The listing builds one solid part. Answer for the finished solid, in the listing's coordinates (mm). A direction names the side the tool comes from. Round coordinates to 2 decimals unless told otherwise and drop trailing zeros. Write each loop counter-clockwise with the first axis right and the second up, starting at its lowest first coordinate (ties: lowest second). Pieces come first, ordered by that corner, then holes. Notation, with made-up numbers: (78, -24) - (118, -24) arc R20 cw to (118, -11) - close; hole circle Ø2 at (-29.5, 42.25). An arc over 180 degrees is marked (long way). Return JSON: item names as keys, results as strings. Group by question number.
(1) Determine the mould class of faces 6 (the cylindrical face through (-3.32, -5.98, -0.03)), 7 (the flat face through (0, -2, -2)), 8 (the cylindrical face through (1.805, -6.618, -0.028)) for opening direction X: +X half, -X half, draft (parallel to the pull), parting line (faces both ways), or undercut.
(2) Each of these flat-tipped pins is pushed along its axis until it touches: pin 1 (1 mm diameter, centred on y = 0.5, z = 0, fed in from +X); pin 2 (1 mm diameter, centred on x = -2.5, z = 1, fed in from -Y); pin 3 (1 mm diameter, centred on y = -2, z = 1, fed in from -X). Where does it stop, or does it pass through?
(3) Which of the six approach directions +Z, -Z, +X, -X, +Y, -Y give full straight-line access (tool end or side, diameter ignored) to faces 1 (the cylindrical face through (4.66, 5.015, -0.028)), 2 (the cylindrical face through (2.6, 6.85, 0.03)), 3 (the cylindrical face through (-5.534, -1.997, 0.028)), 4 (the cylindrical face through (2.822, 5.177, -0.028)), 5 (the cylindrical face through (-0.16, -6.84, -0.03))?
(4) Section A-A, the plane x = -2.75 is taken. Write down the section's boundary in (y, z), then the cut area to 3 significant figures.
(5) Find the intervals of material crossed by line 1 along X through (y, z) = (0, 0.3); line 2 along Y through (x, z) = (-6.5, -1.45); line 3 along X through (y, z) = (5.5, 0.35), in increasing order. Write a range as [from, to].
```python
from build123d import *

# Parameters (mm, degrees)
SKETCH1_R                = 7.326923077
BLANK_DISK_DEPTH         = 2
GEAR_TOOTH_CUT_DEPTH     = 12.107097013
GEAR_START               = -2.000000064
GEAR_TEETH_REVOLVE_DEPTH = 4.000000128
SKETCH4_R                = 0.75
HUB_EXTRUDE_DEPTH        = 0.635
HEX_BORE_CUT_DEPTH       = 12.099256278
HEX_BORE_CUT_DEPTH_BACK  = 12.099256278


# Read off the part's stored shape, not the designer's step: GEAR TEETH REVOLVE
with BuildPart() as part:
    # Sketch1 → BLANK DISK (new, symmetric)
    with BuildSketch(Plane.XY):
        Circle(SKETCH1_R)
    extrude(amount=BLANK_DISK_DEPTH, both=True)

    # Sketch2 → GEAR TOOTH CUT (cut, through all)
    with BuildSketch(Plane.XY.offset(2.000000064)):
        with BuildLine():
            ThreePointArc((-6.69170719, -2.984100644), (-7.114016008, -1.753447463), (-7.311993171, -0.467501495))
            ThreePointArc((-7.311993171, -0.467501495), (-6.820672406, -0.660972702), (-6.303462426, -0.767373077))
            ThreePointArc((-6.303462426, -0.767373077), (-5.834645763, -0.80350314), (-5.364440786, -0.802189535))
            ThreePointArc((-5.364440786, -0.802189535), (-5.140559328, -0.873425337), (-5.015496519, -1.072314102))
            ThreePointArc((-5.015496519, -1.072314102), (-4.979811206, -1.227413224), (-4.939330826, -1.381330469))
            ThreePointArc((-4.939330826, -1.381330469), (-4.957640225, -1.615557309), (-5.122772484, -1.782676381))
            ThreePointArc((-5.122772484, -1.782676381), (-5.539728776, -2.000028389), (-5.938054838, -2.249889939))
            ThreePointArc((-5.938054838, -2.249889939), (-6.346574811, -2.584462254), (-6.69170719, -2.984100644))
        make_face()
    extrude(amount=-GEAR_TOOTH_CUT_DEPTH, mode=Mode.SUBTRACT)

    # GEAR TEETH REVOLVE outline → GEAR TEETH REVOLVE (cut)
    with BuildSketch(Plane.XY.offset(GEAR_START)):
        with BuildLine():
            ThreePointArc((-6.257189634, -3.812004676), (-5.484280674, -4.858648706), (-4.538431736, -5.752081287))
            ThreePointArc((-4.538431736, -5.752081287), (-4.418553413, -5.237828053), (-4.212310448, -4.751730284))
            ThreePointArc((-4.212310448, -4.751730284), (-3.975726688, -4.345377518), (-3.707538741, -3.959152621))
            ThreePointArc((-3.707538741, -3.959152621), (-3.638985493, -3.734435245), (-3.731623965, -3.518528876))
            ThreePointArc((-3.731623965, -3.518528876), (-3.838996472, -3.401054095), (-3.942672404, -3.280304435))
            ThreePointArc((-3.942672404, -3.280304435), (-4.145838239, -3.162316765), (-4.377180353, -3.203283496))
            ThreePointArc((-4.377180353, -3.203283496), (-4.79291572, -3.422961784), (-5.224822737, -3.608840169))
            ThreePointArc((-5.224822737, -3.608840169), (-5.73223615, -3.754986778), (-6.257189634, -3.812004676))
        make_face()
        with BuildLine():
            ThreePointArc((-3.76893936, -6.283223524), (-2.59816273, -6.850792084), (-1.345456266, -7.202329428))
            ThreePointArc((-1.345456266, -7.202329428), (-1.478294676, -6.691270569), (-1.521576498, -6.165006485))
            ThreePointArc((-1.521576498, -6.165006485), (-1.500933528, -5.695253025), (-1.442952554, -5.228634709))
            ThreePointArc((-1.442952554, -5.228634709), (-1.486683039, -4.997799072), (-1.669047026, -4.849674721))
            ThreePointArc((-1.669047026, -4.849674721), (-1.818713911, -4.79555446), (-1.966629555, -4.736816554))
            ThreePointArc((-1.966629555, -4.736816554), (-2.201355572, -4.726759531), (-2.387160652, -4.870543812))
            ThreePointArc((-2.387160652, -4.870543812), (-2.653186447, -5.258261134), (-2.949239125, -5.623565469))
            ThreePointArc((-2.949239125, -5.623565469), (-3.330613673, -5.988778635), (-3.76893936, -6.283223524))
        make_face()
        with BuildLine():
            ThreePointArc((-0.4172705, -7.315031584), (0.883162984, -7.273501556), (2.15574702, -7.002610694))
            ThreePointArc((2.15574702, -7.002610694), (1.800623555, -6.611823636), (1.517732291, -6.165953997))
            ThreePointArc((1.517732291, -6.165953997), (1.317705414, -5.740414699), (1.152196674, -5.300299598))
            ThreePointArc((1.152196674, -5.300299598), (1.006200583, -5.116227361), (0.775888474, -5.069818532))
            ThreePointArc((0.775888474, -5.069818532), (0.618214089, -5.091451091), (0.459944425, -5.108181085))
            ThreePointArc((0.459944425, -5.108181085), (0.247431127, -5.208358653), (0.149728787, -5.422021237))
            ThreePointArc((0.149728787, -5.422021237), (0.094355867, -5.888956227), (0.001979628, -6.349999691))
            ThreePointArc((0.001979628, -6.349999691), (-0.165987742, -6.850613479), (-0.4172705, -7.315031584))
        make_face()
        with BuildLine():
            ThreePointArc((3.029990003, -6.671054064), (4.162166701, -6.029939477), (5.163094643, -5.198678241))
            ThreePointArc((5.163094643, -5.198678241), (4.667040629, -5.017687589), (4.209346902, -4.754355756))
            ThreePointArc((4.209346902, -4.754355756), (3.834473927, -4.470516545), (3.483391529, -4.157729723))
            ThreePointArc((3.483391529, -4.157729723), (3.268575777, -4.062589619), (3.043077274, -4.128528015))
            ThreePointArc((3.043077274, -4.128528015), (2.913516691, -4.220957635), (2.78115068, -4.30932289))
            ThreePointArc((2.78115068, -4.30932289), (2.639534337, -4.496785575), (2.652317164, -4.731378938))
            ThreePointArc((2.652317164, -4.731378938), (2.820282389, -5.170562418), (2.952744873, -5.621725511))
            ThreePointArc((2.952744873, -5.621725511), (3.036663981, -6.143055335), (3.029990003, -6.671054064))
        make_face()
        with BuildLine():
            ThreePointArc((5.783116312, -4.498818453), (6.487668187, -3.404990933), (6.987639506, -2.203791254))
            ThreePointArc((6.987639506, -2.203791254), (6.46429494, -2.274059785), (5.936650867, -2.253591908))
            ThreePointArc((5.936650867, -2.253591908), (5.472810673, -2.176476926), (5.016583365, -2.062674076))
            ThreePointArc((5.016583365, -2.062674076), (4.782159651, -2.078261555), (4.613133744, -2.241441485))
            ThreePointArc((4.613133744, -2.241441485), (4.541367732, -2.383493654), (4.46522883, -2.523250753))
            ThreePointArc((4.46522883, -2.523250753), (4.42695204, -2.755053113), (4.547291643, -2.956834745))
            ThreePointArc((4.547291643, -2.956834745), (4.900116204, -3.267655071), (5.227071851, -3.605581764))
            ThreePointArc((5.227071851, -3.605581764), (5.543652581, -4.028197244), (5.783116312, -4.498818453))
        make_face()
        with BuildLine():
            ThreePointArc((7.211400368, -1.295957751), (7.326923076, 0), (7.211400368, 1.295957751))
            ThreePointArc((7.211400368, 1.295957751), (6.780657183, 0.990527711), (6.303939662, 0.763442688))
            ThreePointArc((6.303939662, 0.763442688), (5.857392449, 0.616167327), (5.400536408, 0.504915345))
            ThreePointArc((5.400536408, 0.504915345), (5.200208381, 0.382171186), (5.126376868, 0.159132278))
            ThreePointArc((5.126376868, 0.159132278), (5.128846154, 0), (5.126376868, -0.159132278))
            ThreePointArc((5.126376868, -0.159132278), (5.200208381, -0.382171186), (5.400536408, -0.504915345))
            ThreePointArc((5.400536408, -0.504915345), (5.857392449, -0.616167327), (6.303939662, -0.763442688))
            ThreePointArc((6.303939662, -0.763442688), (6.780657183, -0.990527711), (7.211400368, -1.295957751))
        make_face()
        with BuildLine():
            ThreePointArc((6.987639507, 2.203791254), (6.487668188, 3.404990933), (5.783116313, 4.498818454))
            ThreePointArc((5.783116313, 4.498818454), (5.543652581, 4.028197244), (5.227071851, 3.605581764))
            ThreePointArc((5.227071851, 3.605581764), (4.900116204, 3.267655071), (4.547291643, 2.956834745))
            ThreePointArc((4.547291643, 2.956834745), (4.42695204, 2.755053113), (4.46522883, 2.523250753))
            ThreePointArc((4.46522883, 2.523250753), (4.541367732, 2.383493654), (4.613133744, 2.241441485))
            ThreePointArc((4.613133744, 2.241441485), (4.782159651, 2.078261555), (5.016583365, 2.062674076))
            ThreePointArc((5.016583365, 2.062674076), (5.472810673, 2.176476926), (5.936650867, 2.253591908))
            ThreePointArc((5.936650867, 2.253591908), (6.46429494, 2.274059785), (6.987639507, 2.203791254))
        make_face()
        with BuildLine():
            ThreePointArc((5.163094645, 5.198678243), (4.162166702, 6.02993948), (3.029990004, 6.671054067))
            ThreePointArc((3.029990004, 6.671054067), (3.036663981, 6.143055335), (2.952744873, 5.621725511))
            ThreePointArc((2.952744873, 5.621725511), (2.820282389, 5.170562418), (2.652317164, 4.731378938))
            ThreePointArc((2.652317164, 4.731378938), (2.639534337, 4.496785575), (2.78115068, 4.30932289))
            ThreePointArc((2.78115068, 4.30932289), (2.913516691, 4.220957635), (3.043077274, 4.128528015))
            ThreePointArc((3.043077274, 4.128528015), (3.268575777, 4.062589619), (3.483391529, 4.157729723))
            ThreePointArc((3.483391529, 4.157729723), (3.834473927, 4.470516545), (4.209346902, 4.754355756))
            ThreePointArc((4.209346902, 4.754355756), (4.667040629, 5.017687589), (5.163094645, 5.198678243))
        make_face()
        with BuildLine():
            ThreePointArc((2.155747021, 7.002610697), (0.883162984, 7.27350156), (-0.4172705, 7.315031588))
            ThreePointArc((-0.4172705, 7.315031588), (-0.165987742, 6.850613479), (0.001979628, 6.349999691))
            ThreePointArc((0.001979628, 6.349999691), (0.094355867, 5.888956227), (0.149728787, 5.422021237))
            ThreePointArc((0.149728787, 5.422021237), (0.247431127, 5.208358653), (0.459944425, 5.108181085))
            ThreePointArc((0.459944425, 5.108181085), (0.618214089, 5.091451091), (0.775888474, 5.069818532))
            ThreePointArc((0.775888474, 5.069818532), (1.006200583, 5.116227361), (1.152196674, 5.300299598))
            ThreePointArc((1.152196674, 5.300299598), (1.317705414, 5.740414699), (1.517732291, 6.165953997))
            ThreePointArc((1.517732291, 6.165953997), (1.800623555, 6.611823636), (2.155747021, 7.002610697))
        make_face()
        with BuildLine():
            ThreePointArc((-1.345456266, 7.202329431), (-2.598162731, 6.850792087), (-3.768939362, 6.283223527))
            ThreePointArc((-3.768939362, 6.283223527), (-3.330613673, 5.988778635), (-2.949239125, 5.623565469))
            ThreePointArc((-2.949239125, 5.623565469), (-2.653186447, 5.258261134), (-2.387160652, 4.870543812))
            ThreePointArc((-2.387160652, 4.870543812), (-2.201355572, 4.726759531), (-1.966629555, 4.736816554))
            ThreePointArc((-1.966629555, 4.736816554), (-1.818713911, 4.79555446), (-1.669047026, 4.849674721))
            ThreePointArc((-1.669047026, 4.849674721), (-1.486683039, 4.997799072), (-1.442952554, 5.228634709))
            ThreePointArc((-1.442952554, 5.228634709), (-1.500933528, 5.695253025), (-1.521576498, 6.165006485))
            ThreePointArc((-1.521576498, 6.165006485), (-1.478294676, 6.691270569), (-1.345456266, 7.202329431))
        make_face()
        with BuildLine():
            ThreePointArc((-4.538431738, 5.752081289), (-5.484280676, 4.858648708), (-6.257189636, 3.812004677))
            ThreePointArc((-6.257189636, 3.812004677), (-5.73223615, 3.754986778), (-5.224822737, 3.608840169))
            ThreePointArc((-5.224822737, 3.608840169), (-4.79291572, 3.422961784), (-4.377180353, 3.203283496))
            ThreePointArc((-4.377180353, 3.203283496), (-4.145838239, 3.162316765), (-3.942672404, 3.280304435))
            ThreePointArc((-3.942672404, 3.280304435), (-3.838996472, 3.401054095), (-3.731623965, 3.518528876))
            ThreePointArc((-3.731623965, 3.518528876), (-3.638985493, 3.734435245), (-3.707538741, 3.959152621))
            ThreePointArc((-3.707538741, 3.959152621), (-3.975726688, 4.345377518), (-4.212310448, 4.751730284))
            ThreePointArc((-4.212310448, 4.751730284), (-4.418553413, 5.237828053), (-4.538431738, 5.752081289))
        make_face()
        with BuildLine():
            ThreePointArc((-5.015496519, 1.072314102), (-4.979811206, 1.227413224), (-4.939330826, 1.381330469))
            ThreePointArc((-4.939330826, 1.381330469), (-4.957640225, 1.61555731), (-5.122772484, 1.782676381))
            ThreePointArc((-5.122772484, 1.782676381), (-5.539728776, 2.000028389), (-5.938054838, 2.249889939))
            ThreePointArc((-5.938054838, 2.249889939), (-6.346574811, 2.584462254), (-6.69170719, 2.984100644))
            ThreePointArc((-6.69170719, 2.984100644), (-7.114016009, 1.753447463), (-7.311993171, 0.467501495))
            ThreePointArc((-7.311993171, 0.467501495), (-6.820672405, 0.660972702), (-6.303462426, 0.767373077))
            ThreePointArc((-6.303462426, 0.767373077), (-5.834645762, 0.80350314), (-5.364440786, 0.802189535))
            ThreePointArc((-5.364440786, 0.802189535), (-5.140559328, 0.873425337), (-5.015496519, 1.072314102))
        make_face()
    extrude(amount=GEAR_TEETH_REVOLVE_DEPTH, mode=Mode.SUBTRACT)

    # Sketch4 → Hub Extrude (add)
    with BuildSketch(Plane.XY.offset(2.000000064)):
        Circle(SKETCH4_R)
    extrude(amount=HUB_EXTRUDE_DEPTH)

    # Sketch3 → HEX BORE CUT (cut, two sides: drawn at the far end of the back side and taken through both)
    with BuildSketch(Plane.XY.offset(2.000000064).offset(-HEX_BORE_CUT_DEPTH_BACK)):
        with BuildLine():
            Line((-1.168931136, -0.94), (1.168931136, -0.94))
            ThreePointArc((1.168931136, -0.94), (0, 1.5), (-1.168931136, -0.94))
        make_face()
    extrude(amount=HEX_BORE_CUT_DEPTH + HEX_BORE_CUT_DEPTH_BACK, mode=Mode.SUBTRACT)


solid = part.part
```
Working result:
{
 "1": {"face 6": "undercut", "face 7": "draft", "face 8": "undercut"},
 "2": {"pin 1": "stops at x = 6.8", "pin 2": "stops at y = -5.68", "pin 3": "stops at x = -6.26"},
 "3": {"face 1": "+Z, -Z, +Y", "face 2": "+Z, -Z, +X, +Y", "face 3": "+Z, -Z, -X", "face 4": "+Z, -Z", "face 5": "+Z, -Z, -Y"},
 "4": {"outline": "(-5.38, -2) - (5.38, -2) - (5.38, 2) - (-5.38, 2) - close", "area": "43.1 mm^2"},
 "5": {"line 1": "x = [-7.33, -1.5], [1.5, 5.13]", "line 2": "y = [-3.38, -2.75], [-0.74, 0.74], [2.75, 3.38]", "line 3": "x = [-4.49, -2.84], [-1.48, 0.14], [1.22, 2.92]"}
}
